```python
from build123d import *

# Parameters (mm, degrees)
EXTRUDE_1_DEPTH     = 15
SKETCH_3_W          = 15
SKETCH_3_H          = 3
EXTRUDE_2_DEPTH     = 15
CUT_EXTRUDE_1_DEPTH = 15
SKETCH_5_W          = 15
SKETCH_5_H          = 38
EXTRUDE_3_DEPTH     = 10
SKETCH_6_W          = 8
SKETCH_6_H          = 32
CUT_EXTRUDE_2_DEPTH = 22
SKETCH_7_W          = 7
SKETCH_7_H          = 22
EXTRUDE_4_DEPTH     = 30
CUT_EXTRUDE_3_DEPTH = 30
CUT_EXTRUDE_4_DEPTH = 30
SKETCH_10_W         = 3.405660377
SKETCH_10_H         = 15
CUT_EXTRUDE_5_DEPTH = 10
CUT_EXTRUDE_6_DEPTH = 10
SKETCH_12_W         = 38
SKETCH_12_H         = 15
EXTRUDE_5_DEPTH     = 4
EXTRUDE_START       = 4
SKETCH_13_W         = 29.594339623
SKETCH_13_H         = 15
EXTRUDE_6_DEPTH     = 4
SKETCH_14_W         = 15
SKETCH_14_H         = 46
EXTRUDE_7_DEPTH     = 4
EXTRUDE_9_DEPTH     = 4


with BuildPart() as part:
    # Sketch 1 → Extrude 1 (new body)
    with BuildSketch(Plane.XY):
        Polygon((13, 0), (0, 0), (0, -3), (8, -3), (8, -35), (0, -35), (0, -38), (13, -38), align=None)
    extrude(amount=EXTRUDE_1_DEPTH)

    # Sketch 3 → Extrude 2 (add)
    with BuildSketch(Plane.ZY):
        with Locations((7.5, -1.5)):
            Rectangle(SKETCH_3_W, SKETCH_3_H)
        with Locations((7.5, -36.5)):
            Rectangle(SKETCH_3_W, SKETCH_3_H)
    extrude(amount=EXTRUDE_2_DEPTH)

    # Sketch 4 → Cut-Extrude 1 (cut)
    with BuildSketch(Plane.XZ.offset(38)):
        with BuildLine():
            Line((-12.170329997, 8.9885069), (3.570652174, 10.948374319))
            ThreePointArc((3.570652174, 10.948374319), (7.475, 7.5), (3.570652174, 4.051625681))
            Line((3.570652174, 4.051625681), (-12.170329997, 6.0114931))
            ThreePointArc((-12.170329997, 6.0114931), (-13.485, 7.5), (-12.170329997, 8.9885069))
        make_face()
    extrude(amount=-CUT_EXTRUDE_1_DEPTH, mode=Mode.SUBTRACT)

    # Sketch 5 → Extrude 3 (add)
    with BuildSketch(Plane(origin=(13, 0, 0), x_dir=(0, 0, -1), z_dir=(1, 0, 0))):
        with Locations((-7.5, -19)):
            Rectangle(SKETCH_5_W, SKETCH_5_H)
    extrude(amount=EXTRUDE_3_DEPTH)

    # Sketch 6 → Cut-Extrude 2 (cut)
    with BuildSketch(Plane.XY.offset(15)):
        with Locations((12, -19)):
            Rectangle(SKETCH_6_W, SKETCH_6_H)
    extrude(amount=-CUT_EXTRUDE_2_DEPTH, mode=Mode.SUBTRACT)

    # Sketch 7 → Extrude 4 (add)
    with BuildSketch(Plane(origin=(0, 0, 0), x_dir=(-1, 0, 0), z_dir=(0, 0, -1))):
        with Locations((-19.5, -19)):
            Rectangle(SKETCH_7_W, SKETCH_7_H)
    extrude(amount=EXTRUDE_4_DEPTH)

    # Sketch 8 → Cut-Extrude 3 (cut)
    with BuildSketch(Plane(origin=(23, 0, 0), x_dir=(0, 0, -1), z_dir=(1, 0, 0))):
        Polygon((0, -8), (30, -12), (30, -8), align=None)
        Polygon((0, -30), (30, -30), (30, -26), align=None)
    extrude(amount=-CUT_EXTRUDE_3_DEPTH, mode=Mode.SUBTRACT)

    # Sketch 9 → Cut-Extrude 4 (cut)
    with BuildSketch(Plane(origin=(23, 0, 0), x_dir=(0, 0, -1), z_dir=(1, 0, 0))):
        Polygon((5.866710017, -12.950612604), (5.866710017, -19), (5.866710017, -23.641237949), (16.631575815, -19), align=None)
    extrude(amount=-CUT_EXTRUDE_4_DEPTH, mode=Mode.SUBTRACT)

    # Sketch 10 → Cut-Extrude 5 (cut)
    with BuildSketch(Plane(origin=(0, 0, 0), x_dir=(1, 0, 0), z_dir=(0, 1, 0))):
        with Locations((-13.297169812, -7.5)):
            Rectangle(SKETCH_10_W, SKETCH_10_H)
    extrude(amount=-CUT_EXTRUDE_5_DEPTH, mode=Mode.SUBTRACT)

    # Sketch 11 → Cut-Extrude 6 (cut)
    with BuildSketch(Plane(origin=(0, 0, 0), x_dir=(1, 0, 0), z_dir=(0, 1, 0))):
        with BuildLine():
            ThreePointArc((-6.594339623, -15), (-10.129873529, -13.535533906), (-11.594339623, -10))
            Line((-11.594339623, -10), (-11.594339623, -15))
            Line((-11.594339623, -15), (-6.594339623, -15))
        make_face()
        with BuildLine():
            Line((-11.594339623, 0), (-11.594339623, -5))
            ThreePointArc((-11.594339623, -5), (-10.129873529, -1.464466094), (-6.594339623, 0))
            Line((-6.594339623, 0), (-11.594339623, 0))
        make_face()
    extrude(amount=-CUT_EXTRUDE_6_DEPTH, mode=Mode.SUBTRACT)

    # Sketch 13 → Extrude 6 (add)
    with BuildSketch(Plane(origin=(0, 0, 0), x_dir=(1, 0, 0), z_dir=(0, 1, 0)).offset(EXTRUDE_START)):
        with BuildLine():
            Line((-6.594339623, 0), (-6.594339623, -15))
            ThreePointArc((-6.594339623, -15), (-10.129873529, -13.535533906), (-11.594339623, -10))
            Line((-11.594339623, -10), (-11.594339623, -5))
            ThreePointArc((-11.594339623, -5), (-10.129873529, -1.464466094), (-6.594339623, 0))
        make_face()
        with Locations((8.202830189, -7.5)):
            Rectangle(SKETCH_13_W, SKETCH_13_H)
    extrude(amount=-EXTRUDE_6_DEPTH)



with BuildPart() as body_2:
    # Sketch 12 → Extrude 5 (new body)
    with BuildSketch(Plane(origin=(0, -38, 0), x_dir=(-1, 0, 0), z_dir=(0, -1, 0))):
        with Locations((-4, -7.5)):
            Rectangle(SKETCH_12_W, SKETCH_12_H)
        with BuildLine():
            ThreePointArc((-3.570652174, -10.948374319), (-7.475, -7.5), (-3.570652174, -4.051625681))
            Line((-3.570652174, -4.051625681), (12.170329997, -6.0114931))
            ThreePointArc((12.170329997, -6.0114931), (13.485, -7.5), (12.170329997, -8.9885069))
            Line((12.170329997, -8.9885069), (-3.570652174, -10.948374319))
        make_face(mode=Mode.SUBTRACT)
    extrude(amount=EXTRUDE_5_DEPTH)


with BuildPart() as part_1:
    add(part.part)

    add(body_2.part)  # Extrude 7 merges body 2
    # Sketch 14 → Extrude 7 (add)
    with BuildSketch(Plane(origin=(23, 0, 0), x_dir=(0, 0, -1), z_dir=(1, 0, 0))):
        with Locations((-7.5, -19)):
            Rectangle(SKETCH_14_W, SKETCH_14_H)
    extrude(amount=EXTRUDE_7_DEPTH)

    # Sketch 15 → Extrude 9 (add)
    with BuildSketch(Plane(origin=(23, 0, 0), x_dir=(0, 0, -1), z_dir=(1, 0, 0))):
        Polygon((0, -8), (0, -30), (30, -26), (30, -12), align=None)
        Polygon((5.866710017, -12.950612604), (5.866710017, -23.641237949), (16.631575815, -19), align=None, mode=Mode.SUBTRACT)
    extrude(amount=EXTRUDE_9_DEPTH)


solid = part_1.part
```
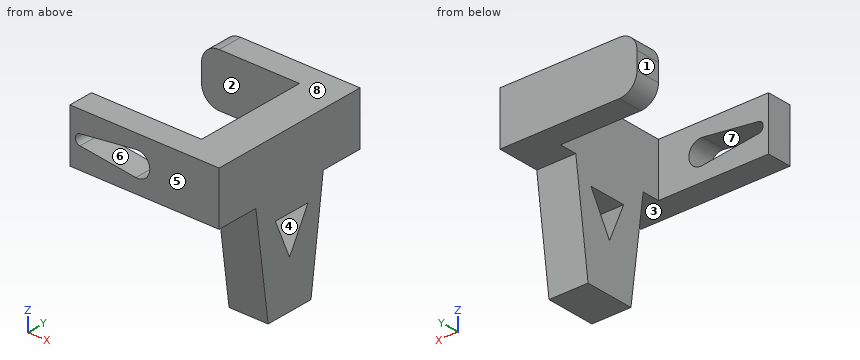
Source: CAD feature listing. Evaluate the final solid. Frame: model axes, mm. Face numbers are marked on the shaded views. A direction names the side the tool comes from. Coordinates: 2 decimals unless noted, no trailing zeros. Write each loop counter-clockwise with the first axis right and the second up, starting at its lowest first coordinate (ties: lowest second). Pieces come first, ordered by that corner, then holes. Notation, with made-up numbers: (-35, 7.25) -> (-21, 7.25) arc R28 cw to (-21, 36.25) -> close; hole circle Ø6 at (-27.5, -23.75). An arc over 180 degrees is marked (long way). Return JSON: item names as keys, results as strings. Group by question number.
1) Contact query for flat-ended pins moving along their axis: P1, Ø12, axis at x = -3.5, y = -30.5, coming from the -Z side; P2, Ø9.5, axis at y = -14, z = 3.5, coming from the -X side; P3, Ø1, axis at y = -7, z = -4.5, coming from the +X side; P4, Ø4, axis at y = 1, z = 7, coming from the -X side. Output: stop coordinate, or through.
2) Ray query, line 1 along X through (y, z) = (-36.25, 7.5) (3 decimals); line 2 along Z through (x, y) = (4, -37.25) (3 decimals); line 3 along Z through (x, y) = (19, -21). Return the intervals inside material, ascending.
3) Section query B-B, the plane x = 23.5. Return loops of the section in (y, z), plus the area to 3 significant figures.
4) Section query D-D, the plane x = -1. Return loops of the section in (y, z), plus the area to 3 significant figures.
5) Mould query, pull axis Z, two halves, no side actions, for the marked faces 5, 6, 7 and 8. Classes: +Z half, -Z half, draft (parallel to the pull), parting line (faces both ways), or undercut.
6) Set-up query: the marked faces 1, 2, 3 and 4. Return all of +Z, -Z, +X, -X, +Y, -Y with unobstructed straight access to the full face (end or side cutting, diameter ignored); none if empty.
7) Section query A-A, the plane z = 7.5. Return loops of the section in (x, y) (3 decimals), plus the area to 3 significant figures.
From the geometry:
{
 "1": {"P1": "z = 0", "P2": "x = 16", "P3": "through", "P4": "x = -11.59"},
 "2": {"line 1": "-15 to -13.485, 7.475 to 27", "line 2": "0 to 4.025, 10.975 to 15", "line 3": "-30 to -11.99, -5.87 to 15"},
 "3": {"outline": "(-42, 0) -> (-30, 0) -> (-26, -30) -> (-12, -30) -> (-8, 0) -> (4, 0) -> (4, 15) -> (-42, 15) -> close; hole (-23.64, -5.87) -> (-19, -16.63) -> (-12.95, -5.87) -> close", "area": "1,170 mm²"},
 "4": {"outline": "(-42, 0) -> (-35, 0) -> (-35, 4.62) -> (-42, 4.62) -> close; (-42, 10.38) -> (-35, 10.38) -> (-35, 15) -> (-42, 15) -> close; (-3, 0) -> (4, 0) -> (4, 15) -> (-3, 15) -> close", "area": "170 mm²"},
 "5": {"face 5": "draft", "face 6": "undercut", "face 7": "undercut", "face 8": "+Z half"},
 "6": {"face 1": "+Z, -Z, -X, +Y", "face 2": "+Z, -Z, -X", "face 3": "-Z, +X, -X, -Y", "face 4": "+X, -X"},
 "7": {"outline": "(-15, -42) -> (-13.485, -42) -> (-13.485, -35) -> (-15, -35) -> close; (-11.594, -3) -> (16, -3) -> (16, -35) -> (7.475, -35) -> (7.475, -42) -> (27, -42) -> (27, 4) -> (-11.594, 4) -> close", "area": "769 mm²"}
}
